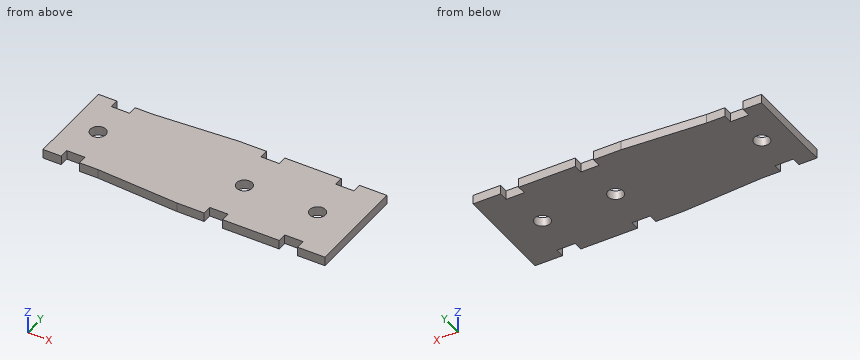
```python
from build123d import *

# Parameters (mm, degrees)
BOSS_EXTRUDE1_DEPTH = 2.5
CUT_EXTRUDE1_REACH  = 111.75
SKETCH2_R           = 4.25


with BuildPart() as part:
    # Sketch1 → Boss-Extrude1 (new, symmetric)
    with BuildSketch(Plane(origin=(0, 0, 0), x_dir=(0, 1, 0), z_dir=(0, 0, 1))):
        Polygon((25, 50), (-25, 50), (-25, 40), (-20, 40), (-20, 30), (-25, 30), (-25, 20), (-28, -25), (-28, -40), (-23, -40), (-23, -50), (-28, -50), (-28, -81), (-23, -81), (-23, -91), (-28, -91), (-28, -106), (28, -106), (28, -91), (23, -91), (23, -81), (28, -81), (28, -50), (23, -50), (23, -40), (28, -40), (28, -25), (25, 20), (25, 30), (20, 30), (20, 40), (25, 40), align=None)
    extrude(amount=BOSS_EXTRUDE1_DEPTH, both=True)

    # Sketch2 → Cut-Extrude1 (cut, up to next)
    with BuildSketch(Plane.XY.offset(2.5), mode=Mode.PRIVATE) as cut_extrude1_sk1:
        with Locations((-35, 0)):
            Circle(SKETCH2_R)
    cut_extrude1_tool1 = extrude(cut_extrude1_sk1.sketch, amount=-CUT_EXTRUDE1_REACH, mode=Mode.PRIVATE) & part.part
    # Sketch2 → Cut-Extrude1 (cut, up to next)
    with BuildSketch(Plane.XY.offset(2.5), mode=Mode.PRIVATE) as cut_extrude1_sk2:
        with Locations((45, 0)):
            Circle(SKETCH2_R)
    cut_extrude1_tool2 = extrude(cut_extrude1_sk2.sketch, amount=-CUT_EXTRUDE1_REACH, mode=Mode.PRIVATE) & part.part
    # Sketch2 → Cut-Extrude1 (cut, up to next)
    with BuildSketch(Plane.XY.offset(2.5), mode=Mode.PRIVATE) as cut_extrude1_sk3:
        with Locations((85, 0)):
            Circle(SKETCH2_R)
    cut_extrude1_tool3 = extrude(cut_extrude1_sk3.sketch, amount=-CUT_EXTRUDE1_REACH, mode=Mode.PRIVATE) & part.part
    add(cut_extrude1_tool1.solids().sort_by_distance((-35, 0, 2.5))[0], mode=Mode.SUBTRACT)
    add(cut_extrude1_tool2.solids().sort_by_distance((45, 0, 2.5))[0], mode=Mode.SUBTRACT)
    add(cut_extrude1_tool3.solids().sort_by_distance((85, 0, 2.5))[0], mode=Mode.SUBTRACT)


solid = part.part
```
Design review of the part built by this model. Coordinates are the model's own, in mm. Round coordinates to 2 decimals unless told otherwise and drop trailing zeros. Write each loop counter-clockwise with the first axis right and the second up, starting at its lowest first coordinate (ties: lowest second). Pieces come first, ordered by that corner, then holes. Notation, with made-up numbers: (78, -29) -> (136, -29) arc R32 cw to (136, -2) -> close; hole circle Ø3 at (51.25, -37.5). An arc over 180 degrees is marked (long way). Answer in a Markdown table with one row per item.
Q1. Take a section at A-A, the plane y = 21.5. State the section outline as (x, z) points, then the cut area to 3 significant figures.
The answers:
| item | result |
|---|---|
| outline | (-50, -2.5) -> (-40, -2.5) -> (-40, 2.5) -> (-50, 2.5) -> close; (-30, -2.5) -> (106, -2.5) -> (106, 2.5) -> (-30, 2.5) -> close |
| area | 730 mm² |
Q2. Take a section at D-D, the plane z = 0.5. Count the separate pieces of the cut face and the enclosed holes in it, then the cut area to 3 significant figures.
The answers:
| item | result |
|---|---|
| separate pieces | 1 |
| enclosed holes | 3 |
| area | 7,950 mm² |
Q3. Take a section at C-C, the plane x = 85. State the section outline as (y, z) points.
The answers:
| item | result |
|---|---|
| outline | (-23, -2.5) -> (-4.25, -2.5) -> (-4.25, 2.5) -> (-23, 2.5) -> close; (4.25, -2.5) -> (23, -2.5) -> (23, 2.5) -> (4.25, 2.5) -> close |
Q4. Take a section at B-B, the plane y = 0. State the section outline as (x, z) points.
The answers:
| item | result |
|---|---|
| outline | (-50, -2.5) -> (-39.25, -2.5) -> (-39.25, 2.5) -> (-50, 2.5) -> close; (-30.75, -2.5) -> (40.75, -2.5) -> (40.75, 2.5) -> (-30.75, 2.5) -> close; (49.25, -2.5) -> (80.75, -2.5) -> (80.75, 2.5) -> (49.25, 2.5) -> close; (89.25, -2.5) -> (106, -2.5) -> (106, 2.5) -> (89.25, 2.5) -> close |
Q5. To check wall thickness, follow L1, parallel to X at y = 23.5, z = 1.55; L2, parallel to X at y = -0.5, z = 0.65; L3, parallel to Y at x = -35, z = -0.1. State the ranges of each line that lie inside material, in increasing order. Write a range as [from, to].
The answers:
| item | result |
|---|---|
| L1 | [-50, -40], [-30, 40], [50, 81], [91, 106] |
| L2 | [-50, -39.22], [-30.78, 40.78], [49.22, 80.78], [89.22, 106] |
| L3 | [-20, -4.25], [4.25, 20] |
Q6. Clearance check with flat-ended pins moving along their axes: pin 1 Ø1.5 at (x, z) = (-3.5, 0) entering from -Y; pin 2 Ø10 at (x, y) = (85, 0) entering from +Z; pin 3 Ø1.5 at (x, z) = (84.5, 0) entering from -Y; pin 4 Ø2.5 at (x, z) = (-27.5, -1) entering from +Y. State where each tip first meets the part, or that it passes through.
The answers:
| item | result |
|---|---|
| pin 1 | y = -26.15 |
| pin 2 | z = 2.5 |
| pin 3 | y = -23 |
| pin 4 | y = 25 |
